Geometry check sheet. Reference: drawing and pictorial views, mm from the part's lowest x, y, z. A direction names the side the tool comes from. Give positions to 0.01 mm unless a question says otherwise; leave off trailing zeros. Order: outer loops, then holes, each group sorted by start corner. A loop starts at its lowest first (then second) coordinate and runs counter-clockwise, first axis right, second up.
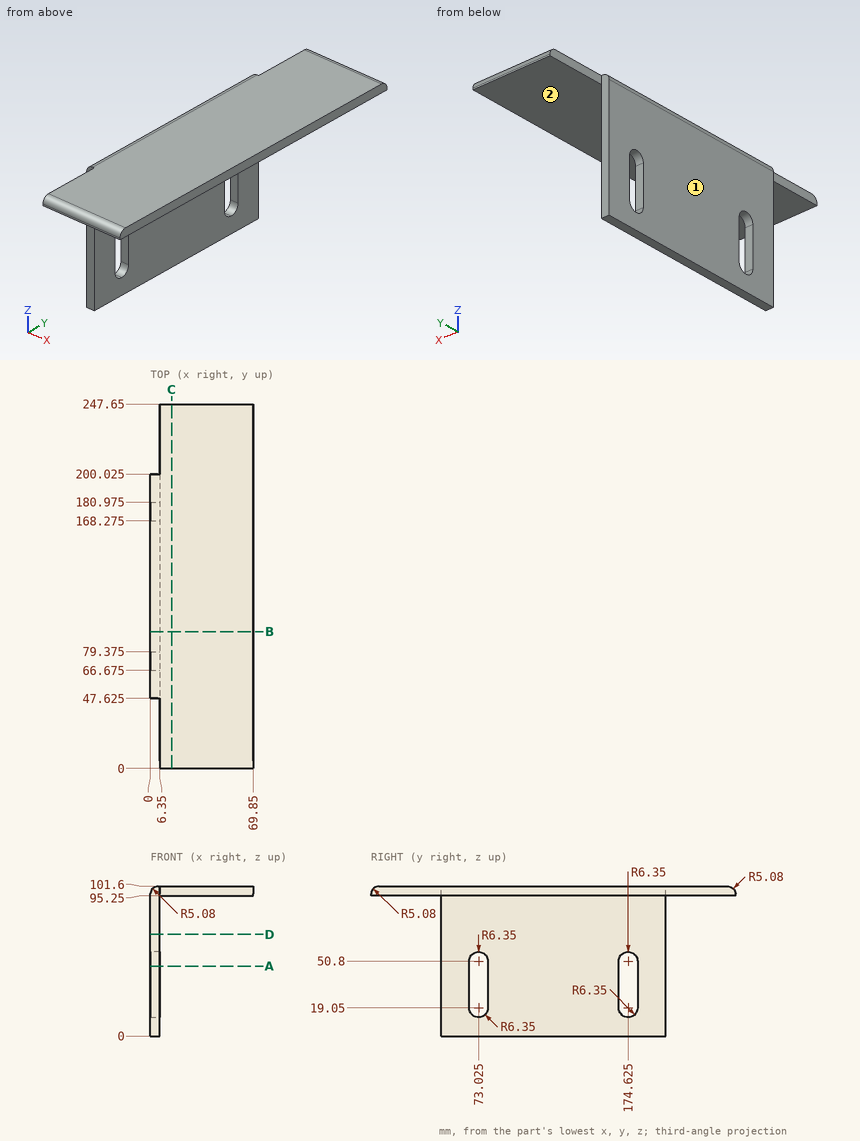
1) Section check D-D, the plane z = 69. Record the cut outline in (x, y) (3 decimals), then the cut area to 3 significant figures.
Recorded:
outline: (0, 47.625) - (6.35, 47.625) - (6.35, 200.025) - (0, 200.025) - close
area: 968 mm2
2) Section check C-C, the plane x = 14.5. Record the cut outline in (y, z), then the cut area to 3 significant figures.
Recorded:
outline: (0, 95.25) - (247.65, 95.25) - (247.65, 96.52) arc R5.08 ccw to (242.57, 101.6) - (5.08, 101.6) arc R5.08 ccw to (0, 96.52) - close
area: 1,560 mm2
3) Depth check by flat-ended pin: pin 1 Ø3 at (x, z) = (3, 29.5) entering from -Y (3 decimals); pin 2 Ø5 at (x, z) = (3.5, 39.5) entering from +Y (3 decimals); pin 3 Ø5 at (y, z) = (30.5, 99.5) entering from -X. Enter the tip coordinate at first touch or a pass-through.
Recorded:
pin 1: stops at y = 47.625
pin 2: stops at y = 200.025
pin 3: stops at x = 6.35
4) Material ranges on L1, parallel to Z at x = 63, y = 149; L2, parallel to X at y = 61, z = 74.5; L3, parallel to Z at x = 6, y = 68, recorded low to high.
Recorded:
L1: z = 95.25 to 101.6
L2: x = 0 to 6.35
L3: z = 0 to 15.17, 54.68 to 101.6
5) Section check B-B, the plane y = 93. Record the cut outline in (x, z).
Recorded:
outline: (0, 0) - (6.35, 0) - (6.35, 95.25) - (69.85, 95.25) - (69.85, 101.6) - (5.08, 101.6) arc R5.08 ccw to (0, 96.52) - close
6) Set-up check for the marked faces 1 and 2: record each of +Z, -Z, +X, -X, +Y, -Y from which the full face is reachable in a straight line by a thin tool's end or side.
Recorded:
face 1: +Z, -Z, -X, +Y, -Y
face 2: -Z, +X, +Y, -Y
7) Section check A-A, the plane z = 47.5. Record the cut outline in (x, y) (3 decimals).
Recorded:
outline: (0, 47.625) - (6.35, 47.625) - (6.35, 66.675) - (0, 66.675) - close; (0, 79.375) - (6.35, 79.375) - (6.35, 168.275) - (0, 168.275) - close; (0, 180.975) - (6.35, 180.975) - (6.35, 200.025) - (0, 200.025) - close
